```python
from build123d import *

# Parameters (mm, degrees)
F0_R     = 44.45
F0_R_2   = 40.64
F1_DEPTH = 6.35
F2_W     = 6.626951
F2_H     = 3.175
F2_W_2   = 3.175
F2_H_2   = 6.626951
F3_DEPTH = 5.08


with BuildPart() as f1:
    # F0 (on Top) → F1 (new body)
    with BuildSketch(Plane.XY):
        Circle(F0_R)
        Circle(F0_R_2, mode=Mode.SUBTRACT)
    extrude(amount=F1_DEPTH)

    # F2 (on face) → F3 (cut)
    with BuildSketch(Plane.XY.offset(6.35)):
        with Locations((-42.241248, 0)):
            Rectangle(F2_W, F2_H)
        Polygon((-44.059319, 11.684578), (-44.765823, 8.589181), (-38.305023, 7.114546), (-37.598519, 10.209942), align=None)
        Polygon((-40.354597, 21.195742), (-41.732178, 18.335165), (-35.761501, 15.459839), (-34.38392, 18.320415), align=None)
        Polygon((-34.626327, 29.644063), (-36.605907, 27.161748), (-31.424748, 23.029911), (-29.445167, 25.512226), align=None)
        Polygon((-27.161748, 36.605907), (-29.644063, 34.626327), (-25.512226, 29.445167), (-23.029911, 31.424748), align=None)
        Polygon((-18.335165, 41.732178), (-21.195742, 40.354597), (-18.320415, 34.38392), (-15.459839, 35.761501), align=None)
        Polygon((-8.589181, 44.765823), (-11.684578, 44.059319), (-10.209942, 37.598519), (-7.114546, 38.305023), align=None)
        with Locations((0, 42.241248)):
            Rectangle(F2_W_2, F2_H_2)
        Polygon((11.684578, 44.059319), (8.589181, 44.765823), (7.114546, 38.305023), (10.209942, 37.598519), align=None)
        Polygon((21.195742, 40.354597), (18.335165, 41.732178), (15.459839, 35.761501), (18.320415, 34.38392), align=None)
        Polygon((29.644063, 34.626327), (27.161748, 36.605907), (23.029911, 31.424748), (25.512226, 29.445167), align=None)
        Polygon((36.605907, 27.161748), (34.626327, 29.644063), (29.445167, 25.512226), (31.424748, 23.029911), align=None)
        Polygon((41.732178, 18.335165), (40.354597, 21.195742), (34.38392, 18.320415), (35.761501, 15.459839), align=None)
        Polygon((44.765823, 8.589181), (44.059319, 11.684578), (37.598519, 10.209942), (38.305023, 7.114546), align=None)
        with Locations((42.241248, 0)):
            Rectangle(F2_W, F2_H)
        Polygon((-44.059319, -11.684578), (-37.598519, -10.209942), (-38.305023, -7.114546), (-44.765823, -8.589181), align=None)
        with Locations((0, -42.241248)):
            Rectangle(F2_W_2, F2_H_2)
        Polygon((21.195742, -40.354597), (18.320415, -34.38392), (15.459839, -35.761501), (18.335165, -41.732178), align=None)
        Polygon((-18.335165, -41.732178), (-15.459839, -35.761501), (-18.320415, -34.38392), (-21.195742, -40.354597), align=None)
        Polygon((-36.605907, -27.161748), (-34.626327, -29.644063), (-29.445167, -25.512226), (-31.424748, -23.029911), align=None)
        Polygon((40.354597, -21.195742), (41.732178, -18.335165), (35.761501, -15.459839), (34.38392, -18.320415), align=None)
        Polygon((27.161748, -36.605907), (29.644063, -34.626327), (25.512226, -29.445167), (23.029911, -31.424748), align=None)
        Polygon((34.626327, -29.644063), (36.605907, -27.161748), (31.424748, -23.029911), (29.445167, -25.512226), align=None)
        Polygon((-27.161748, -36.605907), (-23.029911, -31.424748), (-25.512226, -29.445167), (-29.644063, -34.626327), align=None)
        Polygon((44.765823, -8.589181), (38.305023, -7.114546), (37.598519, -10.209942), (44.059319, -11.684578), align=None)
        Polygon((-8.589181, -44.765823), (-7.114546, -38.305023), (-10.209942, -37.598519), (-11.684578, -44.059319), align=None)
        Polygon((-40.354597, -21.195742), (-34.38392, -18.320415), (-35.761501, -15.459839), (-41.732178, -18.335165), align=None)
        Polygon((8.589181, -44.765823), (11.684578, -44.059319), (10.209942, -37.598519), (7.114546, -38.305023), align=None)
    extrude(amount=-F3_DEPTH, mode=Mode.SUBTRACT)


solid = f1.part
```
The listing builds one solid part. Answer for the finished solid, in the listing's coordinates (mm). A direction names the side the tool comes from. Coordinates: 2 decimals unless noted, no trailing zeros. Write each loop counter-clockwise with the first axis right and the second up, starting at its lowest first coordinate (ties: lowest second). Pieces come first, ordered by that corner, then holes.
Q1. Section C-C, the plane z = 3.25 is taken. Give the number of separate pieces and of enclosed holes in the cut face, then the cut area to 3 significant figures.
Returned:
separate pieces: 28
enclosed holes: 0
area: 680 mm2
Q2. Section A-A, the plane y = 0 is taken. Write down the section's boundary in (x, z), then the cut area to 3 significant figures.
Returned:
outline: (-44.45, 0) - (-40.64, 0) - (-40.64, 1.27) - (-44.45, 1.27) - close; (40.64, 0) - (44.45, 0) - (44.45, 1.27) - (40.64, 1.27) - close
area: 9.68 mm2
Q3. Which of the six approach directions +Z, -Z, +X, -X, +Y, -Y give full straight-line access (tool end or side, diameter ignored) to faces 4 (the flat face through (-39.02, 17.03, 3.85)), 5 (the flat face through (-11.014, 41.122, 3.846)), 6 (the flat face through (-37.592, 19.865, 3.846))?
Returned:
face 4: +Z
face 5: +Z, +Y
face 6: +Z, -X
Q4. Given P1, Ø1.4, axis at x = -19, y = 39.5, coming from the +Z side; P2, Ø5, axis at x = 17.5, y = 39.5, coming from the +Z side; P3, Ø1, axis at x = 26, z = 2.5, coming from the +Y side; P4, Ø1.5, axis at y = 29.5, z = 3.5, coming from the -X side, each flat-ended and moving along its own axis, determine where each tip first touches the part or whether it passes through.
Returned:
P1: stops at z = 1.27
P2: stops at z = 6.35
P3: stops at y = 36.41
P4: stops at x = -33.74
Q5. The mould has two halves that part along Y. Classify faces 1 (the flat face through (9, -41, 1.27)), 2 (the flat face through (11.002, 41.07, 3.846)), 3 (the flat face through (42, -5, 6.35)): released by +Y, released by -Y, zero draft, split by the parting line, or undercut.
Returned:
face 1: undercut
face 2: released by +Y
face 3: zero draft
Q6. Find the intervals of material crossed by line 1 along X through (y, z) = (33, 1.75); line 2 along Z through (x, y) = (-31, -26.5); line 3 along Y through (x, z) = (-25.5, 0.5), in increasing order.
Returned:
line 1: x = -29.78 to -28.35, -24.29 to -23.72, 23.72 to 24.29, 28.35 to 29.78
line 2: z = 0 to 1.27
line 3: y = -36.41 to -31.64, 31.64 to 36.41
